```python
from build123d import *

# Parameters (mm, degrees)
CROSSRECESS_DEPTH = 1.35
DRAFT9_ANGLE      = 30
FILLET5_R         = 0.3
SKETCH10_W        = 0.8
SKETCH10_H        = 2.5


with BuildPart() as part:
    # Sketch1 → Base (revolve)
    with BuildSketch(Plane.XY, mode=Mode.PRIVATE) as base_sk:
        Polygon((10, 2.5), (4.3, 2.5), (2.7, 2.5), (0.75, 4.45), (0, 4.45), (0, 0), (10, 0), align=None)
    revolve(base_sk.sketch.rotate(Axis((4.515812911, 0, 0), (-1, 0, 0)), 90), axis=Axis((4.515812911, 0, 0), (-1, 0, 0)))

    # Sketch6 → CrossRecess (cut)
    with BuildSketch(Plane(origin=(0, 0, 0), x_dir=(0, 0, -1), z_dir=(1, 0, 0))):
        Polygon((0.52, 0.52), (0.52, 2.6), (-0.52, 2.6), (-0.52, 0.52), (-2.6, 0.52), (-2.6, -0.52), (-0.52, -0.52), (-0.52, -2.6), (0.52, -2.6), (0.52, -0.52), (2.6, -0.52), (2.6, 0.52), align=None)
    extrude(amount=CROSSRECESS_DEPTH, mode=Mode.SUBTRACT)

    # Draft9
    draft9_faces = [part.faces().sort_by_distance(p)[0] for p in [
        (0.675, -2.6, 0),
        (0.675, 0, 2.6),
        (0.675, 0, -2.6),
        (0.675, 2.6, 0),
    ]]
    draft(draft9_faces, Plane(origin=(0, 4.45, 0), x_dir=(0, 0, -1), z_dir=(-1, 0, 0)), DRAFT9_ANGLE)

    # Fillet5
    fillet5_edges = [part.edges().sort_by_distance(p)[0] for p in [
        (0.675, 0.52, 0.52),
        (0.675, -0.52, 0.52),
        (0.675, -0.52, -0.52),
        (0.675, 0.52, -0.52),
    ]]
    fillet(fillet5_edges, radius=FILLET5_R)

    # Sketch10 → Revolve2 (revolve)
    with BuildSketch(Plane.XY):
        with Locations((3.1, 1.25)):
            Rectangle(SKETCH10_W, SKETCH10_H)
    revolve(axis=Axis((62.228915663, 0, 0), (-1, 0, 0)))


solid = part.part
```
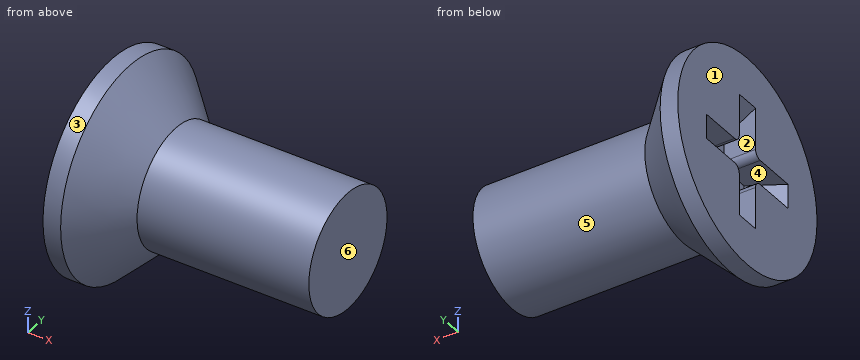
Geometry: final body of the model. Coordinates: model frame, mm. Face numbers are marked on the shaded views. A direction names the side the tool comes from. Coordinates: 2 decimals unless noted, no trailing zeros. Order: outer loops, then holes, each group sorted by start corner. A loop starts at its lowest first (then second) coordinate and runs counter-clockwise, first axis right, second up. Notation, with made-up numbers: (43, -1) -> (48, -1) arc R13 cw to (48, 5) -> close; hole circle Ø3 at (89, -13.5). An arc over 180 degrees is marked (long way). Use CSV: the item, a comma, the result in double quotes.
1) Line query: line 1 (Y direction, x = 1, z = 0.75); line 2 (Y direction, x = 3.25, z = -1.25); line 3 (X direction, y = -3, z = 3.25). Output: solid intervals per line, ascending.
Findings:
line 1,"y = -4.13 to -0.53, 0.53 to 4.13"
line 2,"y = -2.17 to 2.17"
line 3,"x = 0 to 0.78"
2) Access query for the marked faces 4, 5 and 6. Directions: +Z, -Z, +X, -X, +Y, -Y. A direction counts if a zero-diameter tool reaches every point of the face in a straight line with its end or side. Return the directions, or none.
Findings:
face 4,"-X"
face 5,"+X"
face 6,"+Z, -Z, +X, +Y, -Y"
3) Section A-A on z = 0. Output: boundary loops of the cut face in (x, y), then the cut area to 3 significant figures.
Findings:
outline,"(0, -4.45) -> (0.75, -4.45) -> (2.7, -2.5) -> (10, -2.5) -> (10, 2.5) -> (2.7, 2.5) -> (0.75, 4.45) -> (0, 4.45) -> (0, 2.6) -> (1.35, 1.82) -> (1.35, -1.82) -> (0, -2.6) -> close"
area,"50.8 mm^2"
4) Section C-C on x = 3. Output: boundary loops of the cut face in (y, z).
Findings:
outline,"circle Ø5 at (0, 0)"
5) Pin query (flat end, axial travel): pin 1 Ø1 at (x, y) = (2, 2) entering from +Z; pin 2 Ø1.5 at (x, z) = (0.5, 1.5) entering from -Y; pin 3 Ø0.7 at (x, y) = (0.5, -2) entering from +Z. Return the tip coordinate at first contact, or that it passes through.
Findings:
pin 1,"stops at z = 3.19"
pin 2,"stops at y = -4.39"
pin 3,"stops at z = 4.13"
6) Mould query, pull axis Z, two halves, no side actions, for the marked faces 1, 2 and 3. Classes: +Z half, -Z half, draft (parallel to the pull), parting line (faces both ways), or undercut.
Findings:
face 1,"draft"
face 2,"undercut"
face 3,"parting line"
